Geometry check sheet. Reference: the model listing, model coordinates, mm. Round coordinates to 2 decimals unless told otherwise and drop trailing zeros. Write each loop counter-clockwise with the first axis right and the second up, starting at its lowest first coordinate (ties: lowest second). Pieces come first, ordered by that corner, then holes.
from build123d import *

# Parameters (mm, degrees)
F0_W     = 425
F0_H     = 6
F1_DEPTH = 9
F2_R     = 5.25
F3_DEPTH = 17
F5_DEPTH = 15


with BuildPart() as f1:
    # F0 (on Top) → F1 (new body)
    with BuildSketch(Plane.XY):
        with Locations((183.231094, 0)):
            Rectangle(F0_W, F0_H)
    extrude(amount=F1_DEPTH)

    # F2 (on face) → F3 (join)
    with BuildSketch(Plane.YZ.offset(395.731094)):
        with Locations((0, 4.5)):
            Circle(F2_R)
    extrude(amount=F3_DEPTH)

    # F4 (on face) → F5 (cut)
    with BuildSketch(Plane.YZ.offset(412.731094)):
        Polygon((0.954272, 0.572826), (3.878169, 3.362837), (2.923896, 7.290011), (-0.954272, 8.427174), (-3.878169, 5.637163), (-2.923896, 1.709989), align=None)
    extrude(amount=-F5_DEPTH, mode=Mode.SUBTRACT)


solid = f1.part
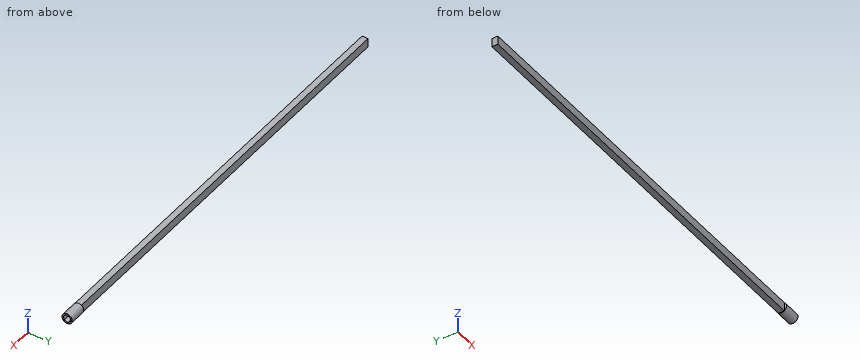
1. Depth check by flat-ended pin: pin 1 Ø0.8 at (y, z) = (0.5, -0.5) entering from -X; pin 2 Ø2 at (y, z) = (-1, 5) entering from +X; pin 3 Ø4.5 at (x, z) = (213, 6) entering from -Y. Enter the tip coordinate at first touch or a pass-through.
2. Scan lines: line 1 along Y through (x, z) = (69, 5); line 2 along Z through (x, y) = (167, -0.75); line 3 along X through (y, z) = (-1.5, 6). Record each from-to range of solid material in increasing order.
3. Section check A-A (x = 48). Record the cut outline in (y, z), plus the area to 3 significant figures.
Results below:
1. pin 1: stops at x = 395.73
1. pin 2: stops at x = 397.73
1. pin 3: stops at y = -3
2. line 1: y = -3 to 3
2. line 2: z = 0 to 9
2. line 3: x = -29.27 to 397.73
3. outline: (-3, 0) - (3, 0) - (3, 9) - (-3, 9) - close
3. area: 54.0 mm2
